from build123d import *

# Parameters (mm, degrees)
SKETCH_1_R      = 10
SKETCH_1_R_2    = 5
EXTRUDE_1_DEPTH = 6.5
SKETCH_2_R      = 1.5
EXTRUDE_2_DEPTH = 2


with BuildPart() as part:
    # 草图1 → 凸台-拉伸1 (new, symmetric)
    with BuildSketch(Plane.XY):
        with Locations(Location((0, 0, 0), (0, 0, 180))):
            Circle(SKETCH_1_R)
        with Locations(Location((0, 0, 0), (0, 0, 180))):
            Circle(SKETCH_1_R_2, mode=Mode.SUBTRACT)
    extrude(amount=EXTRUDE_1_DEPTH, both=True)

    # 草图2 → 凸台-拉伸2 (add, symmetric)
    with BuildSketch(Plane.XY.offset(6.5)):
        with Locations((0, 7.5)):
            Circle(SKETCH_2_R)
        with Locations((7.5, 0)):
            Circle(SKETCH_2_R)
        with Locations((0, -7.5)):
            Circle(SKETCH_2_R)
        with Locations((-7.5, 0)):
            Circle(SKETCH_2_R)
    extrude(amount=EXTRUDE_2_DEPTH, both=True)


solid = part.part
For this review, take the finished solid that the model builds, in its own axes (mm). A direction names the side the tool comes from. Give positions to 0.01 mm unless a question says otherwise; leave off trailing zeros. Loops run counter-clockwise (first coordinate to the right, second up) from the corner with the lowest first, then second, coordinate; pieces in that order, holes last.
Item 1: Take a section at D-D, the plane y = 3.5. State the section outline as (x, z) points.
Item 2: Insertion check: pin 1 (3 mm diameter, centred on y = 2, z = -3, fed in from -X); pin 2 (8 mm diameter, centred on x = 0, y = 0, fed in from +Z); pin 3 (3 mm diameter, centred on y = 4.5, z = 0.5, fed in from -X); pin 4 (5 mm diameter, centred on x = 4, y = -4.5, fed in from +Z). Each pin has a flat end and moves straight along its axis. Give the tip position at first contact, or say it passes through.
Item 3: Tool access review of faces 1 (the flat face through (7, 0, 8.5)), 2 (the cylindrical face through (0, 6, 7)): name each direction out of +Z, -Z, +X, -X, +Y, -Y from which nothing blocks a thin tool from reaching the whole face with its end or side.
Item 4: For line 1 along Y through (x, z) = (0, -2.25); line 2 along X through (y, z) = (-0.25, -4); line 3 along Z through (x, y) = (-3.5, 8.75), list the stretches that pass through material, from the lowest coordinate up.
Item 5: Take a section at A-A, the plane x = 0. State the section outline as (y, z) points, and give its area (3 significant figures).
Item 6: Take a section at C-C, the plane z = -2. State the section outline as (x, y) points, and give its area (3 significant figures).
Item 7: Draft analysis for pull direction X (two halves, no side actions). For faces 3 (the cylindrical face through (6, 0, 7)), 4 (the flat face through (-8, 0, 8.5)), 5 (the cylindrical face through (10, 0, 0)), state which applies: +X half, -X half, draft (parallel to the pull), parting line (faces both ways), or undercut.
Calculated:
1. outline: (-9.37, -6.5) - (-3.57, -6.5) - (-3.57, 6.5) - (-9.37, 6.5) - close; (3.57, -6.5) - (9.37, -6.5) - (9.37, 6.5) - (3.57, 6.5) - close
2. pin 1: stops at x = -9.99
2. pin 2: passes through
2. pin 3: stops at x = -9.54
2. pin 4: stops at z = 6.5
3. face 1: +Z, +X, -X, +Y, -Y
3. face 2: +Z
4. line 1: y = -10 to -5, 5 to 10
4. line 2: x = -10 to -4.99, 4.99 to 10
4. line 3: z = -6.5 to 6.5
5. outline: (-10, -6.5) - (-5, -6.5) - (-5, 6.5) - (-6, 6.5) - (-6, 8.5) - (-9, 8.5) - (-9, 6.5) - (-10, 6.5) - close; (5, -6.5) - (10, -6.5) - (10, 6.5) - (9, 6.5) - (9, 8.5) - (6, 8.5) - (6, 6.5) - (5, 6.5) - close
5. area: 142 mm2
6. outline: circle Ø20 at (0, 0); hole circle Ø10 at (0, 0)
6. area: 236 mm2
7. face 3: undercut
7. face 4: draft
7. face 5: parting line
